```python
from build123d import *

# Parameters (mm, degrees)
F1_DEPTH = 15
F3_DEPTH = 5
F6_D     = 5


with BuildPart() as f1:
    # F0 (on Front) → F1 (new body, symmetric)
    with BuildSketch(Plane.XZ):
        with BuildLine():
            Line((35, 6.25), (-35, 6.25))
            Line((-35, 6.25), (-35, -6.25))
            Line((-35, -6.25), (-25, -6.25))
            ThreePointArc((-25, -6.25), (-17.5, 1.25), (-10, -6.25))
            Line((-10, -6.25), (10, -6.25))
            ThreePointArc((10, -6.25), (17.5, 1.25), (25, -6.25))
            Line((25, -6.25), (35, -6.25))
            Line((35, -6.25), (35, 6.25))
        make_face()
    extrude(amount=F1_DEPTH, both=True)

    # F2 (on face) → F3 (join)
    with BuildSketch(Plane.XZ.offset(15)):
        with BuildLine():
            ThreePointArc((-17.5, 6.25), (-26.338835, 2.588835), (-30, -6.25))
            Line((-30, -6.25), (-25, -6.25))
            ThreePointArc((-25, -6.25), (-17.5, 1.25), (-10, -6.25))
            Line((-10, -6.25), (10, -6.25))
            ThreePointArc((10, -6.25), (17.5, 1.25), (25, -6.25))
            Line((25, -6.25), (30, -6.25))
            ThreePointArc((30, -6.25), (26.338835, 2.588835), (17.5, 6.25))
            Line((17.5, 6.25), (-17.5, 6.25))
        make_face()
    extrude(amount=F3_DEPTH)

    # F4: F1 across plane


with BuildPart() as f1_1:
    add(f1.part)
    add(f1.part.mirror(Plane.XZ))

    # F6 (through all)
    with Locations(Plane(origin=(0, 0, -6.25), x_dir=(1, 0, 0), z_dir=(0, 0, -1))):
        with Locations((-30, 7.5), (-30, -7.5), (0, 15), (0, -15), (30, 7.5), (30, -7.5)):
            Hole(F6_D / 2)


solid = f1_1.part
```
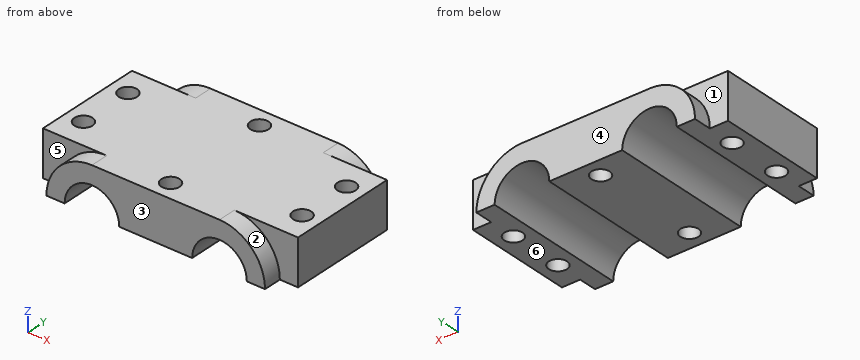
CAD build for the part. Positions are in the model's coordinates, mm. Face numbers are marked on the shaded views. A direction names the side the tool comes from. Coordinates: 2 decimals unless noted, no trailing zeros. Write each loop counter-clockwise with the first axis right and the second up, starting at its lowest first coordinate (ties: lowest second). Pieces come first, ordered by that corner, then holes. Notation, with made-up numbers: (79.5, 80.25) -> (108.5, 80.25) arc R5 cw to (108.5, 84.25) -> close; hole circle Ø10 at (25.5, 25.25). An arc over 180 degrees is marked (long way). Return JSON: item names as keys, results as strings. Group by question number.
Q1. Cut at C-C, the plane z = 0. State how many separate pieces and enclosed holes the cut face has, then the cut area to 3 significant figures.
Q2. Flat gauge pins, fed straight in: pin 1 (6.5 mm diameter, centred on x = 0, y = -15, fed in from +Z); pin 2 (6 mm diameter, centred on x = 17, y = -13, fed in from -Z). Where does each tip first touch, or does it go through?
Q3. Drill centre lines: line 1 (Y direction, x = 0, z = 2); line 2 (Y direction, x = -30, z = 1); line 3 (X direction, y = -14.5, z = 3.75). Where is each one in solid material? Low to high.
Q4. Cut at B-B, the plane y = 9. Give the cut face in (x, z).
Q5. Pull direction Y, two halves, no side cores. Call the marked faces 4, 5 and 6: released by +Y, released by -Y, zero draft, split by the parting line, or undercut.
Q6. Cut at D-D, the plane z = 4.5. Give the cut face in (x, y).
Q7. Which spindle directions (+Z, -Z, +X, -X, +Y, -Y) get a long thin tool onto all of the face, cutting with end or side? Do the marked faces 1, 2 and 3. Say none if no direction does.
Q8. Cut at A-A, the plane x = 0. Give the cut face in (y, z), then the cut area to 3 significant figures.
Returned:
{
 "1": {"separate pieces": "3", "enclosed holes": "6", "area": "1,890 mm2"},
 "2": {"pin 1": "stops at z = 6.25", "pin 2": "stops at z = 0.38"},
 "3": {"line 1": "y = -20 to -17.5, -12.5 to 12.5, 17.5 to 20", "line 2": "y = -15 to -10, -5 to 5, 10 to 15", "line 3": "x = -35 to -2.45, 2.45 to 35"},
 "4": {"outline": "(-35, -6.25) -> (-32, -6.25) -> (-32, 6.25) -> (-35, 6.25) -> close; (-28, -6.25) -> (-25, -6.25) arc R7.5 cw to (-10, -6.25) -> (10, -6.25) arc R7.5 cw to (25, -6.25) -> (28, -6.25) -> (28, 6.25) -> (-28, 6.25) -> close; (32, -6.25) -> (35, -6.25) -> (35, 6.25) -> (32, 6.25) -> close"},
 "5": {"face 4": "released by +Y", "face 5": "released by -Y", "face 6": "zero draft"},
 "6": {"outline": "(-35, -15) -> (-23.88, -15) -> (-23.88, -20) -> (23.88, -20) -> (23.88, -15) -> (35, -15) -> (35, 15) -> (23.88, 15) -> (23.88, 20) -> (-23.88, 20) -> (-23.88, 15) -> (-35, 15) -> close; hole circle Ø5 at (-30, -7.5); hole circle Ø5 at (-30, 7.5); hole circle Ø5 at (0, -15); hole circle Ø5 at (0, 15); hole circle Ø5 at (30, -7.5); hole circle Ø5 at (30, 7.5)"},
 "7": {"face 1": "+Z, -X, +Y", "face 2": "+Z, +X, -Y", "face 3": "+Z, -Z, +X, -X, -Y"},
 "8": {"outline": "(-20, -6.25) -> (-17.5, -6.25) -> (-17.5, 6.25) -> (-20, 6.25) -> close; (-12.5, -6.25) -> (12.5, -6.25) -> (12.5, 6.25) -> (-12.5, 6.25) -> close; (17.5, -6.25) -> (20, -6.25) -> (20, 6.25) -> (17.5, 6.25) -> close", "area": "375 mm2"}
}
